Autodesk Inventor part; units mm, degrees
ref_plane "YZ Plane" through (0, 0, 0) normal (1, 0, 0) x (0, 1, 0)
ref_plane "XZ Plane" through (0, 0, 0) normal (0, 1, 0) x (-1, 0, 0)
ref_plane "XY Plane" through (0, 0, 0) normal (0, 0, 1) x (1, 0, 0)
sketch "Sketch1" plane through (0, 0, 0) normal (0, 1, 0) x (-1, 0, 0)
  circle A0 centre (0, 0) radius 4.25
  circle A1 centre (0, 0) radius 1.75
  dimension "d0" = 8.5
  dimension "d1" = 3.5
extrude "Extrusion1" add sketch "Sketch1" along normal blind 15
sketch "Sketch2" plane through (0, 15, 0) normal (0, 1, 0) x (1, 0, 0)
  line L0 (4.25, 3.75) -> (-4.25, 3.75) construction
  line L1 (-4.25, 3.75) -> (-4.25, -3.75) construction
  line L2 (-4.25, -3.75) -> (4.25, -3.75) construction
  line L3 (4.25, -3.75) -> (4.25, 3.75) construction
  line L4 (4.25, 3.75) -> (-4.25, -3.75) construction
  line L5 (-4.25, 3.75) -> (4.25, -3.75) construction
  line L6 (-4.25, -5.75) -> (4.25, -5.75)
  line L7 (4.25, -5.75) -> (4.25, 5.75)
  line L8 (4.25, 5.75) -> (-4.25, 5.75)
  line L9 (-4.25, 5.75) -> (-4.25, -5.75)
  circle A0 centre (0, 0) radius 1.75
  circle A1 centre (0, 0) radius 1.75
  dimension "d4" = 8.5
  dimension "d5" = 7.5
  dimension "d6" = 11.5
  dimension "d7" = 5.75
extrude "Extrusion2" add sketch "Sketch2" along normal blind 2
sketch "Sketch3" plane through (0, 17, 0) normal (0, 1, 0) x (1, 0, 0)
  line L0 (-4.25, -5.75) -> (4.25, -5.75)
  line L1 (4.25, 5.75) -> (-4.25, 5.75)
  line L2 (-4.25, -5.75) -> (-1.75, -5.75)
  line L3 (-1.75, -5.75) -> (-1.75, 5.75)
  line L4 (-1.75, 5.75) -> (-4.25, 5.75)
  line L5 (-4.25, 5.75) -> (-4.25, -5.75)
  point P0 (0, 0)
  dimension "d10" = 2.5
extrude "Extrusion3" add sketch "Sketch3" along normal blind 6
properties part number "CajonInf"
CAD build for the part. Positions are in the model's coordinates, mm. A direction names the side the tool comes from. Round coordinates to 2 decimals unless told otherwise and drop trailing zeros. Write each loop counter-clockwise with the first axis right and the second up, starting at its lowest first coordinate (ties: lowest second). Pieces come first, ordered by that corner, then holes. Notation, with made-up numbers: (6, 22) -> (51, 22) arc R9 ccw to (51, 33) -> close; hole circle Ø2 at (25.5, 13). An arc over 180 degrees is marked (long way). Answer in a Markdown table with one row per item. Add a question column.
Item 1: Saw through at A-A, the plane y = 7.5. Write the cut outline in (x, z), then the cut area to 3 significant figures.
Item 2: Drop flat-ended pins along their axis: pin 1 Ø3 at (x, z) = (0, 0) entering from +Y; pin 2 Ø1.8 at (y, z) = (18.5, -1.5) entering from +X; pin 3 Ø1.5 at (y, z) = (13.5, 3) entering from -X. Give the stop position or say it passes through.
Item 3: Drill centre lines: line 1 (Z direction, x = 0, y = 11); line 2 (Y direction, x = -0.5, z = 4.5). Where is each one in solid material? Low to high. Write a range as from..to.
Item 4: Saw through at C-C, the plane z = -2.75. Write the cut outline in (x, y).
Item 5: Saw through at D-D, the plane y = 19.5. Write the cut outline in (x, z), then the cut area to 4 significant figures.
Item 6: Which spindle directions (+Z, -Z, +X, -X, +Y, -Y) get a long thin tool onto all of the face, cutting with end or side? Do faces 1 (the face through (-1.75, 20, 0)), 2 (the face through (0, 15, 5)), 3 (the face through (-2.285, 7.395, -3.584)), 4 (the face through (0, 15, -5)). Say none if no direction does.
Findings below:
| question | item | result |
|---|---|---|
| 1 | outline | circle Ø8.5 at (0, 0); hole circle Ø3.5 at (0, 0) |
| 1 | area | 47.1 mm^2 |
| 2 | pin 1 | passes through |
| 2 | pin 2 | stops at x = -1.75 |
| 2 | pin 3 | stops at x = -3.61 |
| 3 | line 1 | z = -4.25..-1.75, 1.75..4.25 |
| 3 | line 2 | y = 15..17 |
| 4 | outline | (-4.25, 15) -> (-3.24, 15) -> (-3.24, 0) -> (3.24, 0) -> (3.24, 15) -> (4.25, 15) -> (4.25, 17) -> (-1.75, 17) -> (-1.75, 23) -> (-4.25, 23) -> close |
| 5 | outline | (-4.25, -5.75) -> (-1.75, -5.75) -> (-1.75, 5.75) -> (-4.25, 5.75) -> close |
| 5 | area | 28.75 mm^2 |
| 6 | face 1 | +Z, -Z, +X, +Y |
| 6 | face 2 | +Z, -Y |
| 6 | face 3 | -Y |
| 6 | face 4 | -Z, -Y |
